Can you work these out from the model? Positions are in its coordinate system, mm. A direction names the side the tool comes from. Give positions to 0.01 mm unless a question says otherwise; leave off trailing zeros. Order: outer loops, then holes, each group sorted by start corner. A loop starts at its lowest first (then second) coordinate and runs counter-clockwise, first axis right, second up. Notation, with made-up numbers: (1.5, 86.5) - (57.5, 86.5) arc R13 cw to (57.5, 90.5) - close; hole circle Ø2 at (-3.5, 16.5). An arc over 180 degrees is marked (long way). One line per question, with ' | ' between items.
```python
from build123d import *

# Parameters (mm, degrees)
F0_R     = 12.7
F2_DEPTH = 38.1
F3_DEPTH = 127
F4_DEPTH = 304.801


with BuildPart() as f2:
    # F0 (on Right) → F2 (new body)
    with BuildSketch(Plane.YZ):
        with BuildLine():
            Line((0, 50.8), (0, 0))
            Line((0, 0), (50.8, 0))
            Line((50.8, 0), (50.8, 16.51))
            Line((50.8, 16.51), (31.75, 16.51))
            Line((31.75, 16.51), (31.75, 29.21))
            Line((31.75, 29.21), (50.8, 29.21))
            Line((50.8, 29.21), (50.8, 38.1))
            Line((50.8, 38.1), (76.2, 38.1))
            Line((76.2, 38.1), (76.2, 29.21))
            Line((76.2, 29.21), (95.25, 29.21))
            Line((95.25, 29.21), (95.25, 16.51))
            Line((95.25, 16.51), (76.2, 16.51))
            Line((76.2, 16.51), (76.2, 0))
            Line((76.2, 0), (127, 0))
            Line((127, 0), (127, 50.8))
            Line((127, 50.8), (111.125, 50.8))
            Line((111.125, 50.8), (84.593426, 90.350173))
            ThreePointArc((84.593426, 90.350173), (63.5, 101.6), (42.406574, 90.350173))
            Line((42.406574, 90.350173), (15.875, 50.8))
            Line((15.875, 50.8), (0, 50.8))
        make_face()
        with Locations((63.5, 76.2)):
            Circle(F0_R, mode=Mode.SUBTRACT)
    extrude(amount=-F2_DEPTH)

    # F1 (on Front) → F3 (join)
    with BuildSketch(Plane.XZ):
        Polygon((0, 0), (0, 38.1), (-273.05, 38.1), (-273.05, 101.6), (-292.019098, 101.6), (-304.8, 87.473746), (-304.8, 0), align=None)
    extrude(amount=-F3_DEPTH)

    # F0 (on Right) → F4 (cut, through all)
    with BuildSketch(Plane.YZ):
        Polygon((50.8, 16.51), (50.8, 0), (76.2, 0), (76.2, 16.51), (95.25, 16.51), (95.25, 29.21), (76.2, 29.21), (76.2, 38.1), (50.8, 38.1), (50.8, 29.21), (31.75, 29.21), (31.75, 16.51), align=None)
    extrude(amount=-F4_DEPTH, mode=Mode.SUBTRACT)


solid = f2.part
```
(1) Will this pin go through, and if not, where does the flat tip stop? pin 1 (9.5 mm diameter, centred on x = -222.5, y = 82, fed in from +Z).
Answer below:
pin 1: z = 38.1
(2) On a 3-axis mill with a long thin cutter (end or side, diameter ignored), from which of +Z, -Z, +X, -X, +Y, -Y can I reach the whole of each face in a straight line? I mean faces 1 (the face through (-18.783, 29.327, 70.852)), 2 (the face through (-19, 119, 50.8)), 3 (the face through (-150, 31.75, 23)), 4 (the face through (-38.1, 63, 63)). Say none if no direction works.
Answer below:
face 1: +Z, +X, -Y | face 2: +Z, +X, +Y | face 3: +X, -X | face 4: +Z, +Y, -Y
(3) Imagine slicing it at D-D (z = 84). List the corners of the cut face in (x, y) for me, and give its area (3 significant figures).
Answer below:
outline: (-304.8, 0) - (-273.05, 0) - (-273.05, 127) - (-304.8, 127) - close; (-38.1, 38.15) - (0, 38.15) - (0, 53.48) - (-38.1, 53.48) - close; (-38.1, 73.52) - (0, 73.52) - (0, 88.85) - (-38.1, 88.85) - close | area: 5,200 mm^2
(4) If we mould it in two halves opening along Z, with no side actions, what happens to faces 5 (the face through (-273.05, 63, 69)), 6 (the face through (-19, 64, 38.1)), 7 (the face through (-282, 63, 101.6)), 8 (the face through (-18.783, 69.36, 64.933))? For each: released by +Z, released by -Z, zero draft, split by the parting line, or undercut.
Answer below:
face 5: zero draft | face 6: released by -Z | face 7: released by +Z | face 8: undercut
(5) Imagine slicing it at A-A (z = 11). List the corners of the cut face in (x, y) for me.
Answer below:
outline: (-304.8, 0) - (0, 0) - (0, 50.8) - (-304.8, 50.8) - close; (-304.8, 76.2) - (0, 76.2) - (0, 127) - (-304.8, 127) - close
(6) Imagine slicing it at C-C (y = 63.5). List the corners of the cut face in (x, z) for me, and give its area (3 significant figures).
Answer below:
outline: (-304.8, 38.1) - (-273.05, 38.1) - (-273.05, 101.6) - (-292.02, 101.6) - (-304.8, 87.47) - close; (-38.1, 38.1) - (0, 38.1) - (0, 63.5) - (-38.1, 63.5) - close; (-38.1, 88.9) - (0, 88.9) - (0, 101.6) - (-38.1, 101.6) - close | area: 3,380 mm^2
(7) Imagine slicing it at B-B (x = -120). List the corners of the cut face in (y, z) for me, and give its area (3 significant figures).
Answer below:
outline: (0, 0) - (50.8, 0) - (50.8, 16.51) - (31.75, 16.51) - (31.75, 29.21) - (50.8, 29.21) - (50.8, 38.1) - (0, 38.1) - close; (76.2, 0) - (127, 0) - (127, 38.1) - (76.2, 38.1) - (76.2, 29.21) - (95.25, 29.21) - (95.25, 16.51) - (76.2, 16.51) - close | area: 3,390 mm^2
(8) If I drill on line 1 (X direction, y = 52, z = 64.5); line 2 (Z direction, x = -10.5, y = 63.5); line 3 (Z direction, x = -247.5, y = 91), over which ranges is the centre line in solid material (lowest first)?
Answer below:
line 1: -304.8 to -273.05, -38.1 to 0 | line 2: 38.1 to 63.5, 88.9 to 101.6 | line 3: 0 to 16.51, 29.21 to 38.1
